```python
from build123d import *

# Parameters (mm, degrees)
SKETCH1_W                = 146
SKETCH1_H                = 50
BOSS_EXTRUDE1_DEPTH      = 26
FILLET1_R                = 4
FILLET2_R                = 10
FILLET3_R                = 1
BOSS_EXTRUDE2_DEPTH      = 18
BOSS_EXTRUDE2_DEPTH_BACK = 10
SKETCH2_R                = 2.5


with BuildPart() as part:
    # Sketch1 → Boss-Extrude1 (new body)
    with BuildSketch(Plane(origin=(0, 0, 0), x_dir=(1, 0, 0), z_dir=(0, 1, 0))):
        Rectangle(SKETCH1_W, SKETCH1_H)
    extrude(amount=BOSS_EXTRUDE1_DEPTH)

    # Fillet1
    fillet1_edges = [part.edges().sort_by_distance(p)[0] for p in [
        (73, 26, 0),
        (73, 0, 0),
    ]]
    fillet(fillet1_edges, radius=FILLET1_R)

    # Fillet2
    fillet2_edges = [part.edges().sort_by_distance(p)[0] for p in [
        (-73, 26, 0),
        (-73, 0, 0),
    ]]
    fillet(fillet2_edges, radius=FILLET2_R)

    # Fillet3
    fillet3_edges = [part.edges().sort_by_distance(p)[0] for p in [
        (73, 13, -25),
        (73, 13, 25),
        (3, 0, -25),
        (3, 26, -25),
        (71.828427125, 24.828427125, -25),
        (71.828427125, 1.171572875, -25),
        (71.828427125, 24.828427125, 25),
        (71.828427125, 1.171572875, 25),
        (-73, 13, 25),
        (-73, 13, -25),
        (3, 0, 25),
        (3, 26, 25),
        (-70.071067812, 23.071067812, 25),
        (-70.071067812, 2.928932188, 25),
        (-70.071067812, 23.071067812, -25),
        (-70.071067812, 2.928932188, -25),
    ]]
    fillet(fillet3_edges, radius=FILLET3_R)

    # Sketch2 → Boss-Extrude2 (add, two sides: drawn at the far end of the back side and taken through both)
    with BuildSketch(Plane.ZY.offset(73).offset(-BOSS_EXTRUDE2_DEPTH_BACK)):
        with Locations((-25.5, 16.5)):
            Circle(SKETCH2_R)
        with Locations((-25.5, 9.5)):
            Circle(SKETCH2_R)
    extrude(amount=BOSS_EXTRUDE2_DEPTH + BOSS_EXTRUDE2_DEPTH_BACK)


solid = part.part
```
CAD build for the part. Positions are in the model's coordinates, mm. A direction names the side the tool comes from. Coordinates: 2 decimals unless noted, no trailing zeros. Write each loop counter-clockwise with the first axis right and the second up, starting at its lowest first coordinate (ties: lowest second). Pieces come first, ordered by that corner, then holes. Notation, with made-up numbers: (2, 13.25) -> (43, 13.25) arc R21 cw to (43, 35.25) -> close; hole circle Ø5 at (-1, -4.5). An arc over 180 degrees is marked (long way). Return JSON: item names as keys, results as strings. Group by question number.
Q1. Which spindle directions (+Z, -Z, +X, -X, +Y, -Y) get a long thin tool onto all of the face, cutting with end or side? Do faces 1 (the face through (-69.99, 23.15, -0.34)), 2 (the face through (-69.99, 2.85, -0.34)), 3 (the face through (73, 13, 0)), 4 (the face through (-63, 17, -26)). Say none if no direction does.
Q2. Cut at A-A, the plane x = -77.5. Give the cut face in (y, z), then the cut area to 3 significant figures.
Q3. Flat gauge pins, fed straight in: pin 1 (6 mm diameter, centred on y = 10, z = -6, fed in from -X); pin 2 (12 mm diameter, centred on x = 9, y = 3.5, fed in from -Z); pin 3 (0.9 mm diameter, centred on y = 17, z = -26.5, fed in from +X). Where does each tip first touch, or does it go through?
Q4. Cut at C-C, the plane x = 36.5. Give the cut face in (y, z), then the cut area to 3 significant figures.
Q5. Cut at B-B, the plane z = 2.5. Give the cut face in (x, y).
Q6. Drill centre lines: line 1 (X direction, y = 14, z = 22); line 2 (Z direction, x = -62, y = 9.5); line 3 (X direction, y = 22, z = -9.5). Where is each one in solid material? Low to high.
Returned:
{
 "1": {"face 1": "+Z, -X, +Y", "face 2": "+Z, -X, -Y", "face 3": "+Z, -Z, +X, +Y, -Y", "face 4": "-Z, +X, +Y, -Y"},
 "2": {"outline": "circle Ø5 at (9.5, -25.5); circle Ø5 at (16.5, -25.5)", "area": "39.3 mm2"},
 "3": {"pin 1": "stops at x = -73", "pin 2": "stops at z = -25", "pin 3": "stops at x = -63"},
 "4": {"outline": "(0, -24) arc R1 ccw to (1, -25) -> (25, -25) arc R1 ccw to (26, -24) -> (26, 24) arc R1 ccw to (25, 25) -> (1, 25) arc R1 ccw to (0, 24) -> close", "area": "1,300 mm2"},
 "5": {"outline": "(-73, 10) arc R10 ccw to (-63, 0) -> (69, 0) arc R4 ccw to (73, 4) -> (73, 22) arc R4 ccw to (69, 26) -> (-63, 26) arc R10 ccw to (-73, 16) -> close"},
 "6": {"line 1": "x = -73 to 73", "line 2": "z = -25 to 25", "line 3": "x = -71 to 73"}
}
